Autodesk Inventor part; units mm, degrees
ref_plane "YZ Plane" through (0, 0, 0) normal (1, 0, 0) x (0, 1, 0)
ref_plane "XZ Plane" through (0, 0, 0) normal (0, 1, 0) x (-1, 0, 0)
ref_plane "XY Plane" through (0, 0, 0) normal (0, 0, 1) x (1, 0, 0)
sketch "Sketch1" plane through (0, 0, 0) normal (0, 0, 1) x (1, 0, 0)
  line L0 (635, 508) -> (635, -508)
  line L1 (635, -508) -> (-635, -508)
  line L2 (-635, -508) -> (-635, 508)
  line L3 (254, 508) -> (254, 127)
  line L4 (254, 127) -> (-254, 127)
  line L5 (-254, 127) -> (-254, 508)
  line L6 (-635, 508) -> (-254, 508)
  line L7 (254, 508) -> (635, 508)
  point P0 (0, 0)
  dimension "d0" = 1270
  dimension "d1" = 1016
extrude "Extrusion1" add sketch "Sketch1" along normal blind 300
properties part number "051665019_11"
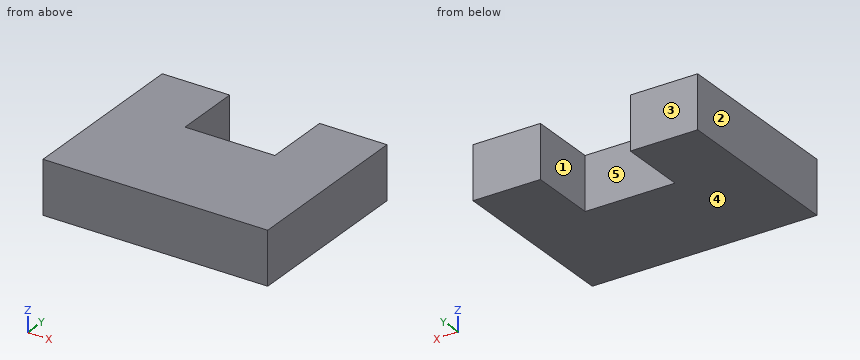
Design review of the part built by this model. Coordinates are the model's own, in mm. Face numbers are marked on the shaded views. A direction names the side the tool comes from. Round coordinates to 2 decimals unless told otherwise and drop trailing zeros. Write each loop counter-clockwise with the first axis right and the second up, starting at its lowest first coordinate (ties: lowest second). Pieces come first, ordered by that corner, then holes. Notation, with made-up numbers: (77, -16) -> (126, -16) arc R22 ccw to (126, 22) -> close; hole circle Ø11 at (-23, 47). An arc over 180 degrees is marked (long way). One line per question, with ' | ' between items.
(1) Draft analysis for pull direction X (two halves, no side actions). For the marked faces 1, 2 and 3, state which applies: released by +X, released by -X, zero draft, split by the parting line, or undercut.
Result sheet:
face 1: undercut | face 2: released by -X | face 3: zero draft
(2) Take a section at A-A, the plane y = 214. State the section outline as (x, z) points.
Result sheet:
outline: (-635, 0) -> (-254, 0) -> (-254, 300) -> (-635, 300) -> close; (254, 0) -> (635, 0) -> (635, 300) -> (254, 300) -> close
(3) Wall thickness on line 1 (Y direction, x = 35, z = 198): over which ranges is the line inside the solid? List them lowest first. Write a range as [from, to].
Result sheet:
line 1: [-508, 127]
(4) Take a section at C-C, the plane x = -204. State the section outline as (y, z) points, and give its area (4 significant figures).
Result sheet:
outline: (-508, 0) -> (127, 0) -> (127, 300) -> (-508, 300) -> close | area: 190,500 mm2
(5) Machinability: for the marked faces 4 and 5, which of the approach directions +Z, -Z, +X, -X, +Y, -Y give a long, thin tool a straight path to every point of the face, cutting with its end or side? Answer none if there is none.
Result sheet:
face 4: -Z, +X, -X, +Y, -Y | face 5: +Z, -Z, +Y
(6) Insertion check: P1, Ø10, axis at x = -448.5, y = 17, coming from the -Z side. The pin has a flat end and moves straight along its axis. Give the tip position at first contact, or say it passes through.
Result sheet:
P1: z = 0
(7) Take a section at B-B, the plane z = 217.5. State the section outline as (x, y) points.
Result sheet:
outline: (-635, -508) -> (635, -508) -> (635, 508) -> (254, 508) -> (254, 127) -> (-254, 127) -> (-254, 508) -> (-635, 508) -> close
